Part model, mm, in its own coordinate system. Round coordinates to 2 decimals unless told otherwise and drop trailing zeros. Write each loop counter-clockwise with the first axis right and the second up, starting at its lowest first coordinate (ties: lowest second). Pieces come first, ordered by that corner, then holes. Notation, with made-up numbers: (12, 39.5) -> (18, 39.5) arc R14 ccw to (18, 63.5) -> close; hole circle Ø5 at (12, -5). An arc over 180 degrees is marked (long way). Return JSON: item names as keys, results as strings. Group by question number.
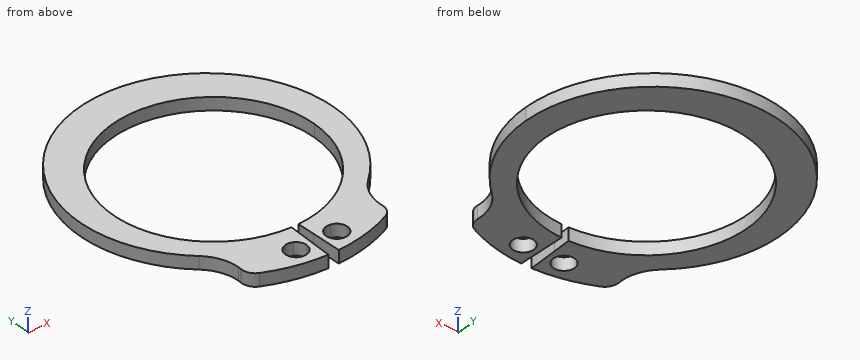
```python
from build123d import *

# Parameters (mm, degrees)
SKETCH3_R           = 1.25
BOSS_EXTRUDE1_DEPTH = 1.2


with BuildPart() as part:
    # Sketch3 → Boss-Extrude1 (new body)
    with BuildSketch(Plane.XY):
        with BuildLine():
            ThreePointArc((9.5, 0), (6.833728103, -6.599254519), (0.331545219, -9.494212857))
            Line((0.331545219, -9.494212857), (0.390890237, -11.193631845))
            ThreePointArc((0.390890237, -11.193631845), (0.917194081, -11.164896783), (1.441728369, -11.113077659))
            ThreePointArc((1.441728369, -11.113077659), (1.771253828, -11.002545946), (2.118708081, -11.011480689))
            ThreePointArc((2.118708081, -11.011480689), (5.247002618, -9.99207874), (7.980846189, -8.161366754))
            ThreePointArc((7.980846189, -8.161366754), (10.949204407, -4.110694744), (12, 0.8))
            ThreePointArc((12, 0.8), (-4.910694694, 11.749204429), (-7.980846271, -8.161366682))
            ThreePointArc((-7.980846271, -8.161366682), (-5.247002667, -9.992078716), (-2.118708081, -11.011480689))
            ThreePointArc((-2.118708081, -11.011480689), (-1.771253828, -11.002545946), (-1.441728369, -11.113077659))
            ThreePointArc((-1.441728369, -11.113077659), (-0.917194081, -11.164896783), (-0.390890237, -11.193631845))
            Line((-0.390890237, -11.193631845), (-0.331545219, -9.494212857))
            ThreePointArc((-0.331545219, -9.494212857), (-6.599254519, 6.833728103), (9.5, 0))
        make_face()
        with BuildLine():
            Line((-0.488592954, -13.991471578), (-0.390890237, -11.193631845))
            ThreePointArc((-0.390890237, -11.193631845), (-0.917194081, -11.164896783), (-1.441728369, -11.113077659))
            ThreePointArc((-1.441728369, -11.113077659), (-1.060032855, -11.480559337), (-0.919665731, -11.991471578))
            ThreePointArc((-0.919665731, -11.991471578), (-2.552499695, -12.765759106), (-2.118708081, -11.011480689))
            ThreePointArc((-2.118708081, -11.011480689), (-5.247002667, -9.992078716), (-7.980846271, -8.161366682))
            ThreePointArc((-7.980846271, -8.161366682), (-6.991393703, -9.511590619), (-6.64112857, -11.148488723))
            ThreePointArc((-6.64112857, -11.148488723), (-6.6440156, -11.300435779), (-6.652672524, -11.452163497))
            ThreePointArc((-6.652672524, -11.452163497), (-5.358796576, -10.297964009), (-4.156280005, -11.547061813))
            ThreePointArc((-4.156280005, -11.547061813), (-4.735472335, -12.601821059), (-5.936307315, -12.679126762))
            ThreePointArc((-5.936307315, -12.679126762), (-3.278779971, -13.610642964), (-0.488592954, -13.991471578))
        make_face()
        with Locations((-5.406280005, -11.547061813)):
            Circle(SKETCH3_R)
        with BuildLine():
            ThreePointArc((1.441728369, -11.113077659), (0.917194081, -11.164896783), (0.390890237, -11.193631845))
            Line((0.390890237, -11.193631845), (0.488592954, -13.991471578))
            ThreePointArc((0.488592954, -13.991471578), (3.278779951, -13.610642969), (5.936307279, -12.67912678))
            ThreePointArc((5.936307279, -12.67912678), (4.326800249, -10.916805153), (6.652672524, -11.452163497))
            ThreePointArc((6.652672524, -11.452163497), (6.931847444, -9.65141373), (7.980846189, -8.161366754))
            ThreePointArc((7.980846189, -8.161366754), (5.247002618, -9.99207874), (2.118708081, -11.011480689))
            ThreePointArc((2.118708081, -11.011480689), (2.693953259, -11.358637615), (2.919665731, -11.991471578))
            ThreePointArc((2.919665731, -11.991471578), (1.40875349, -12.851104454), (1.441728369, -11.113077659))
        make_face()
        with Locations((5.406280005, -11.547061813)):
            Circle(SKETCH3_R)
    extrude(amount=BOSS_EXTRUDE1_DEPTH)


solid = part.part
```
Item 1: Wall check: L1, parallel to X at y = -12.75, z = 0.25; L2, parallel to Y at x = -4, z = 0.5; L3, parallel to X at y = -1.25, z = 0.55. Give the ranges that are in metal, low to high.
Item 2: Cut at D-D (x = 2.5). Write the cut outline in (y, z).
Item 3: Cut at C-C (z = 0.6). Write the cut outline in (x, y).
Item 4: Cut at A-A (y = 6.5). Write the cut outline in (x, z).
Item 5: Cut at B-B (x = -7). Write the cut outline in (y, z), then the cut area to 3 significant figures.
Checks:
{
 "1": {"L1": "x = -5.78 to -2.57, -1.27 to -0.45, 0.45 to 1.27, 2.57 to 5.78", "L2": "y = -13.42 to -8.62, 8.62 to 12.11", "L3": "x = -11.82 to -9.42, 9.42 to 11.82"},
 "2": {"outline": "(-13.77, 0) -> (-12.81, 0) -> (-12.81, 1.2) -> (-13.77, 1.2) -> close; (-11.18, 0) -> (-9.17, 0) -> (-9.17, 1.2) -> (-11.18, 1.2) -> close; (9.17, 0) -> (12.54, 0) -> (12.54, 1.2) -> (9.17, 1.2) -> close"},
 "3": {"outline": "(-7.98, -8.16) arc R4 cw to (-6.65, -11.45) arc R1.25 ccw to (-5.94, -12.68) arc R14 ccw to (-0.49, -13.99) -> (-0.33, -9.49) arc R9.5 cw (long way) to (0.33, -9.49) -> (0.49, -13.99) arc R14 ccw to (5.94, -12.68) arc R1.25 ccw to (6.65, -11.45) arc R4 cw to (7.98, -8.16) arc R12 ccw (long way) to start; hole circle Ø2 at (-1.92, -11.99); hole circle Ø2 at (1.92, -11.99)"},
 "4": {"outline": "(-10.56, 0) -> (-6.93, 0) -> (-6.93, 1.2) -> (-10.56, 1.2) -> close; (6.93, 0) -> (10.56, 0) -> (10.56, 1.2) -> (6.93, 1.2) -> close"},
 "5": {"outline": "(-9.49, 0) -> (-6.42, 0) -> (-6.42, 1.2) -> (-9.49, 1.2) -> close; (6.42, 0) -> (10.55, 0) -> (10.55, 1.2) -> (6.42, 1.2) -> close", "area": "8.63 mm2"}
}
